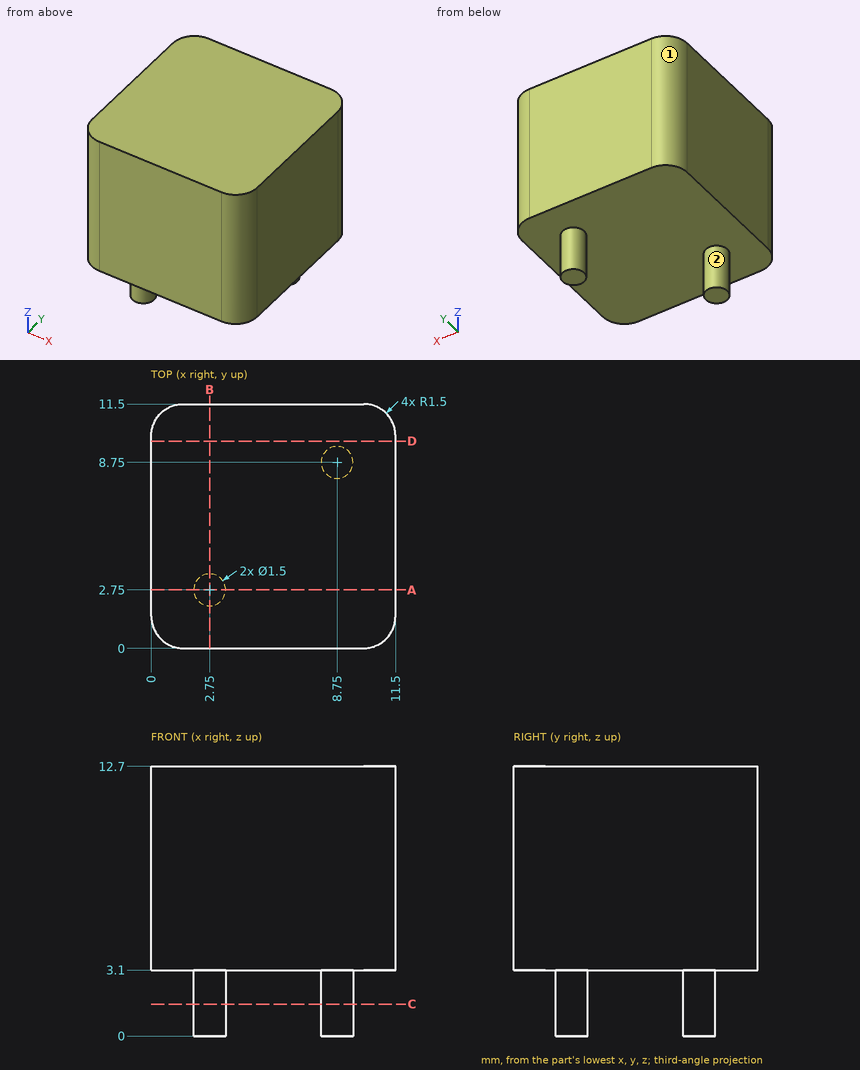
Check sheet for the drawn part. Datum: minimum x, y, z corner. Units: mm. A direction names the side the tool comes from. Coordinates: 2 decimals unless noted, no trailing zeros. Loops run counter-clockwise (first coordinate to the right, second up) from the corner with the lowest first, then second, coordinate; pieces in that order, holes last. Notation, with made-up numbers: (-9, 79) -> (-2, 79) arc R19 cw to (-2, 107) -> close; hole circle Ø3 at (-3.75, -24). An arc over 180 degrees is marked (long way). Answer as a JSON object with one key per item and string values. Group by question number.
Item 1: Sectioned sample at D-D on y = 9.75. Record the boundary of the cut face in (x, z), plus the area to 3 significant figures.
Item 2: Sectioned sample at A-A on y = 2.75. Record the boundary of the cut face in (x, z), plus the area to 3 significant figures.
Item 3: Tool access check on the marked faces 1 and 2. Record the directions out of +Z, -Z, +X, -X, +Y, -Y that give a thin tool (end or side, any length) a straight path to the whole face; none if there is none.
Item 4: Scan lines: probe 1 along Z at (x, y) = (1.75, 2.25); probe 2 along X at (y, z) = (10.25, 10). Record each from-to range of solid material in increasing order.
Item 5: Depth check by flat-ended pin: pin 1 (1 mm diameter, centred on x = 4.5, y = 2, fed in from -Z). Enter the tip coordinate at first touch or a pass-through.
Item 6: Sectioned sample at C-C on z = 1.5. Record the boundary of the cut face in (x, y).
Evaluation:
{
 "1": {"outline": "(0, 3.1) -> (11.5, 3.1) -> (11.5, 12.7) -> (0, 12.7) -> close", "area": "110 mm²"},
 "2": {"outline": "(0, 3.1) -> (2, 3.1) -> (2, 0) -> (3.5, 0) -> (3.5, 3.1) -> (11.5, 3.1) -> (11.5, 12.7) -> (0, 12.7) -> close", "area": "115 mm²"},
 "3": {"face 1": "+Z, -Z, -X, +Y", "face 2": "-Z"},
 "4": {"probe 1": "z = 3.1 to 12.7", "probe 2": "x = 0.02 to 11.48"},
 "5": {"pin 1": "stops at z = 3.1"},
 "6": {"outline": "circle Ø1.5 at (2.75, 2.75); circle Ø1.5 at (8.75, 8.75)"}
}
